Could you check a few things on this model? Use its own coordinates, in mm. Face numbers are marked on the shaded views. A direction names the side the tool comes from. Give positions to 0.01 mm unless a question says otherwise; leave off trailing zeros. Loops run counter-clockwise (first coordinate to the right, second up) from the corner with the lowest first, then second, coordinate; pieces in that order, holes last. Notation, with made-up numbers: (65.5, 73) - (78.5, 73) arc R25 cw to (78.5, 86) - close; hole circle Ø1 at (77.5, 59). An arc over 180 degrees is marked (long way). One line per item, written item: value. Start each with the question number.
Q1. I want a section at A-A (z = 13). Please give me the cut outline in (x, y).
Q2. For the marked faces 1, 2, 3 and 4, which set-ups out of +Z, -Z, +X, -X, +Y, -Y let a thin tool reach every point of the face, with its end or its side?
Q3. I want a section at B-B (y = 6). Please give me the cut outline in (x, z).
Q4. If I drill on line 1 (X direction, y = 17, z = -2); line 2 (Y direction, x = 1.5, z = -1); line 3 (X direction, y = 36.5, z = -4), over which ranges is the centre line in solid material (lowest first)? Write a range as from..to.
Q5. I want a section at D-D (x = 39). Please give me the cut outline in (y, z).
Q6. I'm going to push flat-ended pins straight in: P1, Ø7.5, axis at y = 17.5, z = 3.5, coming from the +X side; P2, Ø1, axis at x = 38.5, y = 21, coming from the +Z side; P3, Ø1.8, axis at x = 36.5, y = 20.5, coming from the -Z side. Where does each tip first touch, or does it pass through?
Q7. I want a section at C-C (x = -46). Please give me the cut outline in (y, z), then the cut area to 3 significant figures.
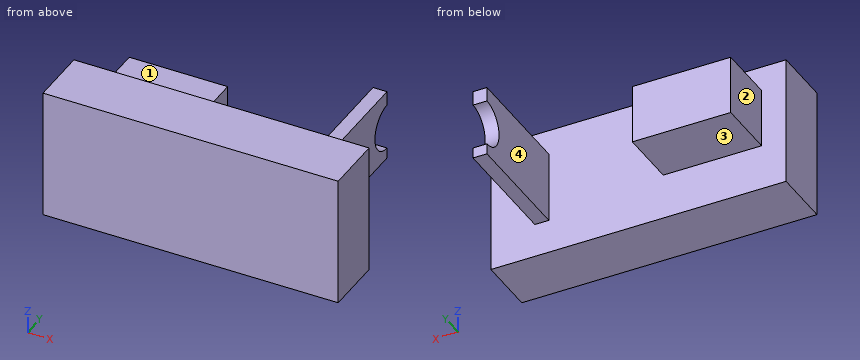
```python
from build123d import *

# Parameters (mm, degrees)
F0_W          = 41.900944
F0_H          = 25.259434
F0_W_2        = 5.943396
F0_H_2        = 30.311321
F0_W_3        = 125.702835
F0_H_3        = 55.570757
F1_DEPTH      = 25
F2_DEPTH      = 25
F2_DEPTH_BACK = 25
F3_DEPTH      = 25
F3_DEPTH_BACK = 50
F5_DEPTH      = 106.982136


with BuildPart() as f1:
    # F0 (on Front) → F1 (new body)
    with BuildSketch(Plane.XZ):
        with Locations((-34.76887, 2.971698)):
            Rectangle(F0_W, F0_H)
        with Locations((37.889149, 0.445754)):
            Rectangle(F0_W_2, F0_H_2)
        with Locations((-3.268871, -1.485849)):
            Rectangle(F0_W_3, F0_H_3)
        with Locations((-34.76887, 2.971698)):
            Rectangle(F0_W, F0_H, mode=Mode.SUBTRACT)
        with Locations((37.889149, 0.445754)):
            Rectangle(F0_W_2, F0_H_2, mode=Mode.SUBTRACT)
    extrude(amount=F1_DEPTH)

    # F0 (on Front) → F2 (join, two sides)
    with BuildSketch(Plane.XZ) as f2_sk:
        with Locations((-34.76887, 2.971698)):
            Rectangle(F0_W, F0_H)
    extrude(amount=F2_DEPTH)
    extrude(f2_sk.sketch, amount=-F2_DEPTH_BACK)

    # F0 (on Front) → F3 (join, two sides)
    with BuildSketch(Plane.XZ) as f3_sk:
        with Locations((37.889149, 0.445754)):
            Rectangle(F0_W_2, F0_H_2)
    extrude(amount=F3_DEPTH)
    extrude(f3_sk.sketch, amount=-F3_DEPTH_BACK)

    # F4 (on face) → F5 (cut, through all)
    with BuildSketch(Plane.YZ.offset(40.860847)):
        with BuildLine():
            Line((50, -10.152427), (50, 9.467568))
            ThreePointArc((50, 9.467568), (40.252312, -0.34243), (50, -10.152427))
        make_face()
    extrude(amount=-F5_DEPTH, mode=Mode.SUBTRACT)


solid = f1.part
```
Worked answers:
1. outline: (-66.12, -25) - (59.58, -25) - (59.58, 0) - (40.86, 0) - (40.86, 50) - (34.92, 50) - (34.92, 0) - (-13.82, 0) - (-13.82, 25) - (-55.72, 25) - (-55.72, 0) - (-66.12, 0) - close
2. face 1: +Z, +X, -X, +Y
2. face 2: +Z, -Z, -X, +Y
2. face 3: -Z, -X, +Y
2. face 4: +Z, -Z, +Y
3. outline: (-55.72, -9.66) - (-13.82, -9.66) - (-13.82, 15.6) - (-55.72, 15.6) - close; (34.92, -14.71) - (40.86, -14.71) - (40.86, 15.6) - (34.92, 15.6) - close
4. line 1: x = -55.72..-13.82, 34.92..40.86
4. line 2: y = -25..0
4. line 3: x = 34.92..40.86
5. outline: (-25, -29.27) - (0, -29.27) - (0, -14.71) - (50, -14.71) - (50, -10.15) arc R9.81 cw to (50, 9.47) - (50, 15.6) - (0, 15.6) - (0, 26.3) - (-25, 26.3) - close
6. P1: stops at x = 40.86
6. P2: stops at z = 15.6
6. P3: stops at z = -14.71
7. outline: (-25, -29.27) - (0, -29.27) - (0, -9.66) - (25, -9.66) - (25, 15.6) - (0, 15.6) - (0, 26.3) - (-25, 26.3) - close
7. area: 2,020 mm²
